For this review, take the finished solid that the model builds, in its own axes (mm). A direction names the side the tool comes from. Round coordinates to 2 decimals unless told otherwise and drop trailing zeros. Write each loop counter-clockwise with the first axis right and the second up, starting at its lowest first coordinate (ties: lowest second). Pieces come first, ordered by that corner, then holes. Notation, with made-up numbers: M 30,-28 L 45,-28 A21 cw 45,-19 Z; hole C 40,-35.5 d6. An arc over 180 degrees is marked long. Use one line per item in the form item = value. Start each with the question number.
Item 1: Add section C-C (z = 11). State the section outline as (x, y) points.
Item 2: For faces 1 (the cylindrical face through (3.47, -32.14, -15.62)), 2 (the cylindrical face through (-37.3, -53.6, -34.7)), 3 (the flat face through (23, -15, -23)), list the 3-axis set-ups (+Z, -Z, +X, -X, +Y, -Y) from which the entire face can be reached by the end or side of a thin tool; tool diameter is ignored.
Item 3: For line 1 (Z direction, x = -34.8, y = -49.5); line 2 (Z direction, x = -34, y = -52); line 3 (Z direction, x = 0, y = -59.2), list the stretches that pass through material, from the lowest coordinate up. Write a range as [from, to].
Item 4: Add section B-B (x = -2.5). State the section outline as (y, z) points, and give its area (3 significant figures).
Item 5: For P1, Ø25, axis at x = 11.5, z = -5.5, coming from the +Y side; P2, Ø8, axis at x = -34.8, z = 34.8, coming from the +Y side; P3, Ø5.5, axis at x = -22.98, z = 22.98, coming from the +Y side; P4, Ø1, axis at x = 15, y = -29.5, coming from the +Z side, all flat-tipped, find the tip position at first contact; note any pin that passes through.
Item 6: Draft analysis for pull direction X (two halves, no side actions). For faces 4 (the flat face through (-1, -46, -41.25)), 5 (the flat face through (41.25, -46, -1)), 6 (the cylindrical face through (-25.842, -7.395, -22.08)), state which applies: released by +X, released by -X, zero draft, split by the parting line, or undercut.
Item 7: Add section D-D (y = -27.5). State the section outline as (x, z) points.
Item 8: Add section A-A (y = -56). State the section outline as (x, z) points.
from build123d import *

# Parameters (mm, degrees)
F0_R      = 40
F1_DEPTH  = 30.5
F2_W      = 82.500003
F2_H      = 82.5
F3_DEPTH  = 30.5
F4_R      = 16
F5_DEPTH  = 61.001
F6_R      = 36.5
F7_DEPTH  = 3
F8_R      = 25
F9_DEPTH  = 7
F10_R     = 2.5
F11_DEPTH = 15
F12_R     = 3
F13_DEPTH = 15


with BuildPart() as f1:
    # F0 (on Front) → F1 (new body)
    with BuildSketch(Plane.XZ):
        Circle(F0_R)
    extrude(amount=F1_DEPTH)

    # F2 (on face) → F3 (join)
    with BuildSketch(Plane.XZ.offset(30.5)):
        with Locations((-1e-06, 0)):
            Rectangle(F2_W, F2_H)
    extrude(amount=F3_DEPTH)

    # F4 (on face) → F5 (cut, through all)
    with BuildSketch(Plane(origin=(0, 0, 0), x_dir=(-1, 0, 0), z_dir=(0, 1, 0))):
        Circle(F4_R)
    extrude(amount=-F5_DEPTH, mode=Mode.SUBTRACT)

    # F6 (on face) → F7 (cut)
    with BuildSketch(Plane.XZ.offset(61)):
        Circle(F6_R)
    extrude(amount=-F7_DEPTH, mode=Mode.SUBTRACT)

    # F8 (on face) → F9 (cut)
    with BuildSketch(Plane(origin=(0, 0, 0), x_dir=(-1, 0, 0), z_dir=(0, 1, 0))):
        Circle(F8_R)
    extrude(amount=-F9_DEPTH, mode=Mode.SUBTRACT)

    # F10 (on face) → F11 (cut)
    with BuildSketch(Plane.XZ.offset(61)):
        with Locations((-34.8, 34.8)):
            Circle(F10_R)
        with Locations((34.8, 34.8)):
            Circle(F10_R)
        with Locations((34.8, -34.8)):
            Circle(F10_R)
        with Locations((-34.8, -34.8)):
            Circle(F10_R)
    extrude(amount=-F11_DEPTH, mode=Mode.SUBTRACT)

    # F12 (on face) → F13 (cut)
    with BuildSketch(Plane(origin=(0, 0, 0), x_dir=(-1, 0, 0), z_dir=(0, 1, 0))):
        with Locations((-22.98097, 22.98097)):
            Circle(F12_R)
        with Locations((-22.98097, -22.98097)):
            Circle(F12_R)
        with Locations((22.98097, -22.98097)):
            Circle(F12_R)
        with Locations((22.98097, 22.98097)):
            Circle(F12_R)
    extrude(amount=-F13_DEPTH, mode=Mode.SUBTRACT)


solid = f1.part
Calculated:
q1.outline = M -41.25,-61 L -34.8,-61 L -34.8,-58 L -11.62,-58 L -11.62,-7 L -22.45,-7 L -22.45,0 L -38.46,0 L -38.46,-30.5 L -41.25,-30.5 Z; M 11.62,-58 L 34.8,-58 L 34.8,-61 L 41.25,-61 L 41.25,-30.5 L 38.46,-30.5 L 38.46,0 L 22.45,0 L 22.45,-7 L 11.62,-7 Z
q2.face_1 = +Y, -Y
q2.face_2 = -Y
q2.face_3 = +Y
q3.line_1 = [-41.25, -37.3], [-32.3, 32.3], [37.3, 41.25]
q3.line_2 = [-41.25, -37.17], [-32.43, 32.43], [37.17, 41.25]
q3.line_3 = [-41.25, -36.5], [36.5, 41.25]
q4.outline = M -61,-41.25 L -30.5,-41.25 L -30.5,-39.92 L 0,-39.92 L 0,-24.87 L -7,-24.87 L -7,-15.8 L -58,-15.8 L -58,-36.41 L -61,-36.41 Z; M -61,36.41 L -58,36.41 L -58,15.8 L -7,15.8 L -7,24.87 L 0,24.87 L 0,39.92 L -30.5,39.92 L -30.5,41.25 L -61,41.25 Z
q4.area = 2,770 mm^2
q5.P1 = 0
q5.P2 = -30.5
q5.P3 = -15
q5.P4 = 37.28
q6.face_4 = zero draft
q6.face_5 = released by +X
q6.face_6 = undercut
q7.outline = C 0,0 d80; hole C 0,0 d32
q8.outline = M -41.25,-41.25 L 41.25,-41.25 L 41.25,41.25 L -41.25,41.25 Z; hole C -34.8,-34.8 d5; hole C -34.8,34.8 d5; hole C 0,0 d32; hole C 34.8,-34.8 d5; hole C 34.8,34.8 d5
